```python
from build123d import *

# Parameters (mm, degrees)
F0_W     = 50.8
F0_H     = 50.8
F1_DEPTH = 50.8
F2_R     = 12.7
F3_DEPTH = 50.8
F4_W     = 22.8882213071
F4_H     = 22.126223892
F5_DEPTH = 12.7
F6_R     = 12.7
F7_DEPTH = 12.7


with BuildPart() as f1:
    # F0 (on Front) → F1 (new body)
    with BuildSketch(Plane.XZ):
        with Locations((25.4, -25.4)):
            Rectangle(F0_W, F0_H)
    extrude(amount=F1_DEPTH)

    # F2 (on face) → F3 (cut)
    with BuildSketch(Plane(origin=(0, 0, 0), x_dir=(-1, 0, 0), z_dir=(0, 1, 0))):
        with Locations((-25.4, -25.4)):
            Circle(F2_R)
    extrude(amount=-F3_DEPTH, mode=Mode.SUBTRACT)

    # F4 (on face) → F5 (join)
    with BuildSketch(Plane(origin=(0, 0, 0), x_dir=(0, -1, 0), z_dir=(-1, 0, 0))):
        with Locations((26.6558893465, -23.763111946)):
            Rectangle(F4_W, F4_H)
    extrude(amount=F5_DEPTH)

    # F6 (on face) → F7 (join)
    with BuildSketch(Plane.YZ.offset(50.8)):
        with Locations((-25.4, -25.4)):
            Circle(F6_R)
    extrude(amount=F7_DEPTH)


solid = f1.part
```
Here's how the part is built. I have some questions about the finished solid (model axes, mm). A direction names the side the tool comes from. Give positions to 0.01 mm unless a question says otherwise; leave off trailing zeros. Order: outer loops, then holes, each group sorted by start corner. A loop starts at its lowest first (then second) coordinate and runs counter-clockwise, first axis right, second up. Notation, with made-up numbers: (15.25, 54.5) -> (22.25, 54.5) arc R29 ccw to (22.25, 77.5) -> close; hole circle Ø3 at (54, 8). An arc over 180 degrees is marked (long way). Use CSV: the item, a comma, the result in double quotes. Start each with the question number.
Item 1: Thinking about a two-plate mould opening in X: for faces 6 (the flat face through (63.5, -26, -25)), 7 (the cylindrical face through (28.15, -25.04, -37.8)), 8 (the flat face through (-6, -26, -12.7)), which applies, pulls with the +X half, pulls with the -X half, needs draft (parallel to the pull), parting line crosses it, or undercut?
Item 2: Suppose I cut it at D-D (y = -9). List the corners of the cut face in (x, z) for me, and give its area (3 significant figures).
Item 3: On a 3-axis mill with a long thin cutter (end or side, diameter ignored), from which of +Z, -Z, +X, -X, +Y, -Y can I reach the whole of each face in a straight line? I mean faces 1 (the flat face through (25, -25, 0)), 2 (the flat face through (-6, -15.212, -24)), 3 (the flat face through (-6, -38.1, -24)), 4 (the flat face through (50.8, -13.8, -31.4)), 5 (the flat face through (-6, -26, -34.826)). Say none if no direction works.
Item 4: Suppose I cut it at B-B (z = -25.4). List the corners of the cut face in (x, y) for me, and give its area (3 significant figures).
Item 5: Suppose I cut it at A-A (x = 25.4). List the corners of the cut face in (y, z) for me.
Item 6: If I drill on probe 1 along Z at (x, y) = (25, -11); probe 2 along X at (y, z) = (-37.5, -40); probe 3 along Z at (x, y) = (-6, -24), over which ranges is the centre line in solid material (lowest first)? Write a range as [from, to].
Item 7: I'm going to push flat-ended pins straight in: P1, Ø14, axis at x = -8.5, y = -30, coming from the -Z side; P2, Ø4, axis at x = -5, z = -19, coming from the +Y side; P3, Ø2, axis at x = -2.5, z = -25, coming from the -Y side. Where does each tip first touch, or does it pass through?
Item 8: Suppose I cut it at C-C (y = -25.4). List the corners of the cut face in (x, z) for me.
Answer block:
1,face 6,"pulls with the +X half"
1,face 7,"undercut"
1,face 8,"needs draft"
2,outline,"(0, -50.8) -> (50.8, -50.8) -> (50.8, 0) -> (0, 0) -> close; hole circle Ø25.4 at (25.4, -25.4)"
2,area,"2,070 mm^2"
3,face 1,"+Z, +X, -X, +Y, -Y"
3,face 2,"+Z, -Z, -X, +Y"
3,face 3,"+Z, -Z, -X, -Y"
3,face 4,"+X"
3,face 5,"-Z, -X, +Y, -Y"
4,outline,"(-12.7, -38.1) -> (0, -38.1) -> (0, -50.8) -> (12.7, -50.8) -> (12.7, 0) -> (0, 0) -> (0, -15.21) -> (-12.7, -15.21) -> close; (38.1, -50.8) -> (50.8, -50.8) -> (50.8, -38.1) -> (63.5, -38.1) -> (63.5, -12.7) -> (50.8, -12.7) -> (50.8, 0) -> (38.1, 0) -> close"
4,area,"1,900 mm^2"
5,outline,"(-50.8, -50.8) -> (0, -50.8) -> (0, -38.1) -> (-50.8, -38.1) -> close; (-50.8, -12.7) -> (0, -12.7) -> (0, 0) -> (-50.8, 0) -> close"
6,probe 1,"z = [-50.8, -38.09], [-12.71, 0]"
6,probe 2,"x = [0, 50.8]"
6,probe 3,"z = [-34.83, -12.7]"
7,P1,"stops at z = -34.83"
7,P2,"stops at y = -15.21"
7,P3,"stops at y = -38.1"
8,outline,"(-12.7, -34.83) -> (0, -34.83) -> (0, -50.8) -> (50.8, -50.8) -> (50.8, -38.1) -> (63.5, -38.1) -> (63.5, -12.7) -> (50.8, -12.7) -> (50.8, 0) -> (0, 0) -> (0, -12.7) -> (-12.7, -12.7) -> close; hole circle Ø25.4 at (25.4, -25.4)"
